from build123d import *

# Parameters (mm, degrees)
BOSS_EXTRUDE1_DEPTH = 2.4
SKETCH2_R           = 0.125
BOSS_EXTRUDE2_DEPTH = 36


with BuildPart() as part:
    # Sketch1 → Boss-Extrude1 (new body)
    with BuildSketch(Plane(origin=(0, 0, 0), x_dir=(1, 0, 0), z_dir=(0, 1, 0))):
        with BuildLine():
            Line((-2.15, 1.275735082), (-2.15, -1.275735082))
            ThreePointArc((-2.15, -1.275735082), (0, -2.5), (2.15, -1.275735082))
            Line((2.15, -1.275735082), (2.15, 1.275735082))
            ThreePointArc((2.15, 1.275735082), (0, 2.5), (-2.15, 1.275735082))
        make_face()
    extrude(amount=BOSS_EXTRUDE1_DEPTH)

    # Sketch2 → Boss-Extrude2 (add)
    with BuildSketch(Plane(origin=(0, 0, 0), x_dir=(1, 0, 0), z_dir=(0, 1, 0))):
        with Locations((0, 1.7)):
            Circle(SKETCH2_R)
        with Locations((0, -1.7)):
            Circle(SKETCH2_R)
    extrude(amount=-BOSS_EXTRUDE2_DEPTH)


solid = part.part
Check sheet for the modelled part. Datum: model origin and axes. Units: mm. Give positions to 0.01 mm unless a question says otherwise; leave off trailing zeros. Write each loop counter-clockwise with the first axis right and the second up, starting at its lowest first coordinate (ties: lowest second). Pieces come first, ordered by that corner, then holes. Notation, with made-up numbers: (84.25, 9.5) -> (112.25, 9.5) arc R34 ccw to (112.25, 46.5) -> close; hole circle Ø6 at (-38.75, -18). An arc over 180 degrees is marked (long way). Use one line per item in the form item = value. Start each with the question number.
1. Thickness scan on line 1 along Y through (x, z) = (1.3, 0.85); line 2 along X through (y, z) = (-18.5, 1.75). Record the ranges inside material, lowest first. Write a range as from..to.
2. Section check B-B (z = 0.25). Record the cut outline in (x, y), and give its area (3 significant figures).
3. Section check A-A (y = -1). Record the cut outline in (x, z) (3 decimals), and give its area (3 significant figures).
4. Section check C-C (x = -1.4). Record the cut outline in (y, z).
Conclusion:
q1.line_1 = 0..2.4
q1.line_2 = -0.11..0.11
q2.outline = (-2.15, 0) -> (2.15, 0) -> (2.15, 2.4) -> (-2.15, 2.4) -> close
q2.area = 10.3 mm²
q3.outline = circle Ø0.25 at (0, -1.7); circle Ø0.25 at (0, 1.7)
q3.area = 0.0982 mm²
q4.outline = (0, -2.07) -> (2.4, -2.07) -> (2.4, 2.07) -> (0, 2.07) -> close
